Input: part model. Units: mm. Frame: model coordinates. Face numbers are marked on the shaded views. A direction names the side the tool comes from. Coordinates: 2 decimals unless noted, no trailing zeros. Write each loop counter-clockwise with the first axis right and the second up, starting at its lowest first coordinate (ties: lowest second). Pieces come first, ordered by that corner, then holes. Notation, with made-up numbers: (29.5, 86.5) -> (69.5, 86.5) arc R16 ccw to (69.5, 90.5) -> close; hole circle Ø7 at (59.5, 19). An arc over 180 degrees is marked (long way). Use one line per item in the form item = value. Start each with the question number.
(1) Ray query, line 1 along Z through (x, y) = (40, 4.75); line 2 along Y through (x, z) = (24.5, 19). Return the intervals inside material, ascending.
(2) Cut plane D-D on x = 6.5. Return the cut outline in (y, z).
(3) First-contact query: pin 1 (6 mm diameter, centred on x = 40, z = 0, fed in from +Y); pin 2 (11.5 mm diameter, centred on y = 80, z = 0, fed in from -X); pin 3 (11.5 mm diameter, centred on x = 80, z = 0, fed in from +Y); pin 4 (8 mm diameter, centred on y = 71, z = -10.5, fed in from +X). Flat tips, straight axial feed; report the tip coordinate or a pass-through.
(4) Cut plane C-C on z = -25.5. Return the cut outline in (x, y).
(5) Cut plane A-A on y = 80. Return the cut outline in (x, z).
(6) Set-up query: the marked faces 4 and 5. Return all of +Z, -Z, +X, -X, +Y, -Y with unobstructed straight access to the full face (end or side cutting, diameter ignored); none if empty.
(7) Pull-direction query (Y, two-part tool) for the marked faces 1, 2 and 3; classes: released by +Y, released by -Y, zero draft, split by the parting line, or undercut.
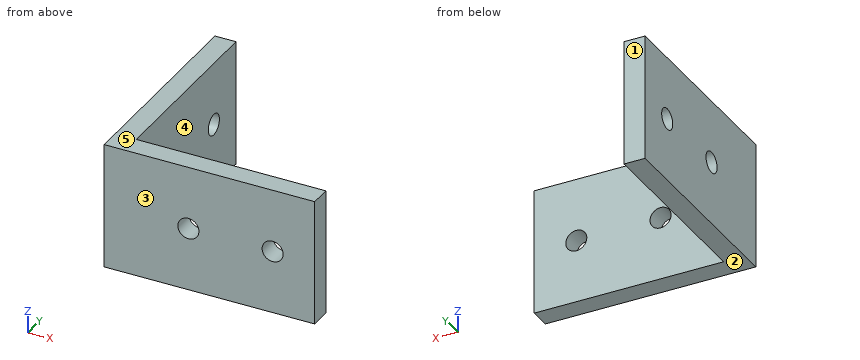
```python
from build123d import *

# Parameters (mm, degrees)
BOSS_EXTRUDE1_DEPTH = 30
SKETCH2_R           = 5
CUT_EXTRUDE1_DEPTH  = 11
SKETCH3_R           = 5
CUT_EXTRUDE2_DEPTH  = 11


with BuildPart() as part:
    # Sketch1 → Boss-Extrude1 (new body, symmetric)
    with BuildSketch(Plane.XY):
        Polygon((0, 0), (0, 100), (10, 100), (10, 10), (100, 10), (100, 0), align=None)
    extrude(amount=BOSS_EXTRUDE1_DEPTH, both=True)

    # Sketch2 → Cut-Extrude1 (cut, through all)
    with BuildSketch(Plane(origin=(10, 0, 0), x_dir=(0, 0, -1), z_dir=(1, 0, 0))):
        with Locations((0, 40)):
            Circle(SKETCH2_R)
        with Locations((0, 80)):
            Circle(SKETCH2_R)
    extrude(amount=-CUT_EXTRUDE1_DEPTH, mode=Mode.SUBTRACT)

    # Sketch3 → Cut-Extrude2 (cut, through all)
    with BuildSketch(Plane(origin=(0, 10, 0), x_dir=(0, 0, -1), z_dir=(0, 1, 0))):
        with Locations((0, -80)):
            Circle(SKETCH3_R)
        with Locations((0, -40)):
            Circle(SKETCH3_R)
    extrude(amount=-CUT_EXTRUDE2_DEPTH, mode=Mode.SUBTRACT)


solid = part.part
```
Values:
q1.line_1 = -30 to -5, 5 to 30
q1.line_2 = 0 to 10
q2.outline = (0, -30) -> (100, -30) -> (100, 30) -> (0, 30) -> close; hole circle Ø10 at (40, 0); hole circle Ø10 at (80, 0)
q3.pin_1 = through
q3.pin_2 = 0
q3.pin_3 = 10
q3.pin_4 = 10
q4.outline = (0, 0) -> (100, 0) -> (100, 10) -> (10, 10) -> (10, 100) -> (0, 100) -> close
q5.outline = (0, -30) -> (10, -30) -> (10, -5) -> (0, -5) -> close; (0, 5) -> (10, 5) -> (10, 30) -> (0, 30) -> close
q6.face_4 = +Z, -Z, +X, +Y
q6.face_5 = +Z, +X, -X, +Y, -Y
q7.face_1 = released by +Y
q7.face_2 = zero draft
q7.face_3 = released by -Y
